from build123d import *

# Parameters (mm, degrees)
SKETCH1_R           = 5.1
BOSS_EXTRUDE1_DEPTH = 10
BOSS_EXTRUDE3_DEPTH = 10
BOSS_EXTRUDE4_DEPTH = 10
CUT_EXTRUDE1_REACH  = 12
SKETCH7_R           = 2.5
CUT_EXTRUDE4_REACH  = 37


with BuildPart() as part:
    # Sketch1 → Boss-Extrude1 (new body)
    with BuildSketch(Plane.XY):
        Polygon((-10, -10), (-10, -15), (10, -15), (10, -10), (10, 10), (-10, 10), align=None)
        Circle(SKETCH1_R, mode=Mode.SUBTRACT)
    extrude(amount=BOSS_EXTRUDE1_DEPTH)

    # Sketch4 → Boss-Extrude3 (add)
    with BuildSketch(Plane.XZ.offset(15)):
        Polygon((-10, 10), (-10, 0), (10, 0), (10, 10), (14.5, 35), (14.5, 40), (-14.5, 40), (-14.5, 35), align=None)
    extrude(amount=BOSS_EXTRUDE3_DEPTH)

    # Sketch6 → Boss-Extrude4 (add)
    with BuildSketch(Plane(origin=(0, -15, 0), x_dir=(1, 0, 0), z_dir=(0, 1, 0))):
        Polygon((0, -35), (10.323759005, -24.676240995), (34.153257531, -48.505739521), (13.505739521, -69.153257531), (-10.323759005, -45.323759005), (-14.5, -40), (-5, -40), align=None)
    extrude(amount=-BOSS_EXTRUDE4_DEPTH)

    # Sketch7 → Cut-Extrude1 (cut, up to next)
    with BuildSketch(Plane(origin=(0, -15, 0), x_dir=(1, 0, 0), z_dir=(0, 1, 0)), mode=Mode.PRIVATE) as cut_extrude1_sk1:
        with Locations((15.432605499, -60.756364505)):
            Circle(SKETCH7_R)
    cut_extrude1_tool1 = extrude(cut_extrude1_sk1.sketch, amount=-CUT_EXTRUDE1_REACH, mode=Mode.PRIVATE) & part.part
    add(cut_extrude1_tool1.solids().sort_by_distance((15.432605, -15, 60.756365))[0], mode=Mode.SUBTRACT)
    # Sketch7 → Cut-Extrude1 (cut, up to next)
    with BuildSketch(Plane(origin=(0, -15, 0), x_dir=(1, 0, 0), z_dir=(0, 1, 0)), mode=Mode.PRIVATE) as cut_extrude1_sk2:
        with Locations((25.756364505, -50.432605499)):
            Circle(SKETCH7_R)
    cut_extrude1_tool2 = extrude(cut_extrude1_sk2.sketch, amount=-CUT_EXTRUDE1_REACH, mode=Mode.PRIVATE) & part.part
    add(cut_extrude1_tool2.solids().sort_by_distance((25.756365, -15, 50.432605))[0], mode=Mode.SUBTRACT)

    # Sketch8 → Cut-Extrude4 (cut, up to next)
    with BuildSketch(Plane.XZ.offset(25), mode=Mode.PRIVATE) as cut_extrude4_sk1:
        Polygon((10, 10), (10, 24.352481989), (13.150544827, 27.503026816), align=None)
    cut_extrude4_tool1 = extrude(cut_extrude4_sk1.sketch, amount=-CUT_EXTRUDE4_REACH, mode=Mode.PRIVATE) & part.part
    add(cut_extrude4_tool1.solids().sort_by_distance((11.050182, -25, 20.618503))[0], mode=Mode.SUBTRACT)
    # Sketch8 → Cut-Extrude4 (cut, up to next)
    with BuildSketch(Plane.XZ.offset(25), mode=Mode.PRIVATE) as cut_extrude4_sk2:
        Polygon((-14.5, 40), (-14.5, 35), (-10, 10), (-10, 45.647518011), (-10.323759005, 45.323759005), align=None)
    cut_extrude4_tool2 = extrude(cut_extrude4_sk2.sketch, amount=-CUT_EXTRUDE4_REACH, mode=Mode.PRIVATE) & part.part
    add(cut_extrude4_tool2.solids().sort_by_distance((-11.684358, -25, 31.470679))[0], mode=Mode.SUBTRACT)


solid = part.part
Work out the finished part from the listing and answer in its coordinate system (mm). A direction names the side the tool comes from. Give positions to 0.01 mm unless a question says otherwise; leave off trailing zeros. Write each loop counter-clockwise with the first axis right and the second up, starting at its lowest first coordinate (ties: lowest second). Pieces come first, ordered by that corner, then holes.
Q1. The part is cut by section D-D on y = -16. Give the vertices of the cut face in (x, z), and give its area (3 significant figures).
Answer:
outline: (-10, 0) - (10, 0) - (10, 24.35) - (34.15, 48.51) - (13.51, 69.15) - (-10, 45.65) - close; hole circle Ø5 at (15.43, 60.76); hole circle Ø5 at (25.76, 50.43)
area: 1,640 mm2
Q2. For a pull along Z with two mould halves and no side action, classify faces 4 (the face through (0, -7, 0)), 5 (the face through (25.214, -19.93, 52.873)), 6 (the face through (7, -15, 39)) as released by +Z, released by -Z, zero draft, split by the parting line, or undercut.
Answer:
face 4: released by -Z
face 5: undercut
face 6: zero draft
Q3. The part is cut by section A-A on y = 0. Give the vertices of the cut face in (x, z), and give its area (3 significant figures).
Answer:
outline: (-10, 0) - (-5.1, 0) - (-5.1, 10) - (-10, 10) - close; (5.1, 0) - (10, 0) - (10, 10) - (5.1, 10) - close
area: 98.0 mm2
Q4. The part is cut by section C-C on x = 0. Give the vertices of the cut face in (y, z).
Answer:
outline: (-25, 0) - (-5.1, 0) - (-5.1, 10) - (-15, 10) - (-15, 55.65) - (-25, 55.65) - close; (5.1, 0) - (10, 0) - (10, 10) - (5.1, 10) - close
Q5. Straight lines are drawn through the part: L1, parallel to Y at x = 4.5, z = 57.5; L2, parallel to X at y = -20, z = 10; L3, parallel to Z at x = 8, y = 0. For each, find the intervals that lie inside material, in ascending order.
Answer:
L1: y = -25 to -15
L2: x = -10 to 10
L3: z = 0 to 10
Q6. The part is cut by section B-B on x = 24. Give the vertices of the cut face in (y, z).
Answer:
outline: (-25, 38.35) - (-15, 38.35) - (-15, 48.65) - (-25, 48.65) - close; (-25, 52.21) - (-15, 52.21) - (-15, 58.66) - (-25, 58.66) - close
Q7. A tool of negligible diameter and unlimited length cuts with its end or side. For faces 1 (the face through (-2, -5, 10)), 2 (the face through (7, -25, 35)), 3 (the face through (10, -12, 9)), from which of +Z, -Z, +X, -X, +Y, -Y can it reach the whole face along a straight path? Write none if from no direction.
Answer:
face 1: +Z, +X, -X, +Y
face 2: +Z, -Z, +X, -X, -Y
face 3: -Z, +X, +Y, -Y
Q8. Given pin 1 (7.5 mm diameter, centred on y = -4.5, z = 8, fed in from +X); pin 2 (8 mm diameter, centred on x = -5, z = 53, fed in from +Y); pin 3 (3 mm diameter, centred on x = -3, y = -16, fed in from -Z); pin 4 (6 mm diameter, centred on x = -3, y = -5, fed in from +Z), each flat-ended and moving along its own axis, determine where each tip first touches the part or whether it passes through.
Answer:
pin 1: stops at x = 10
pin 2: stops at y = -15
pin 3: stops at z = 0
pin 4: stops at z = 10
